Design review of the part shown in the three views and the two pictorial views. Dimensions are in mm from the part's minimum x, y and z. A direction names the side the tool comes from. Round coordinates to 2 decimals unless told otherwise and drop trailing zeros. Order: outer loops, then holes, each group sorted by start corner. A loop starts at its lowest first (then second) coordinate and runs counter-clockwise, first axis right, second up. Notation, with made-up numbers: (39, 85.25) - (93, 85.25) arc R20 cw to (93, 122.25) - close; hole circle Ø10 at (-11, 61). An arc over 180 degrees is marked (long way). Use CSV: the item, a comma, the result in double quotes.
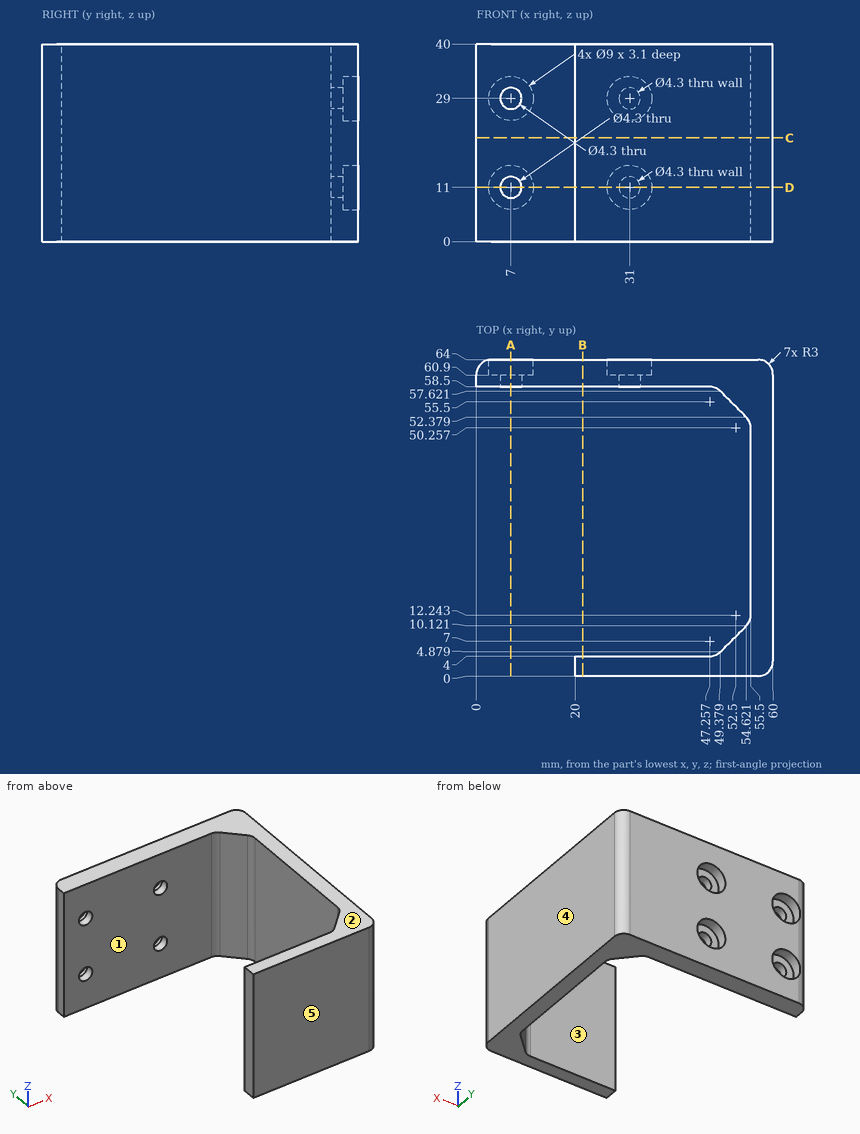
1) Insertion check: pin 1 Ø10 at (x, y) = (17.5, 54) entering from -Z; pin 2 Ø2.5 at (x, z) = (29.5, 10.5) entering from +Y; pin 3 Ø5 at (x, z) = (7, 11) entering from -Y; pin 4 Ø3 at (y, z) = (1.5, 26) entering from -X. Each pin has a flat end and moves straight along its axis. Give the tip position at first contact, or say it passes through.
Data:
pin 1,"stops at z = 0"
pin 2,"stops at y = 60.9"
pin 3,"stops at y = 58.5"
pin 4,"stops at x = 20"
2) We need section D-D (z = 11). Give the number of separate pieces and of enclosed holes in the cut face, then the cut area to 3 significant figures.
Data:
separate pieces,"3"
enclosed holes,"0"
area,"703 mm2"
3) The part is to be moulded in two halves that separate along Y. For the marked faces 3, 4 and 5, say which applies: +Y half, -Y half, draft (parallel to the pull), parting line (faces both ways), or undercut.
Data:
face 3,"undercut"
face 4,"draft"
face 5,"-Y half"
4) For the marked faces 1 and 2, list the 3-axis set-ups (+Z, -Z, +X, -X, +Y, -Y) from which the entire face can be reached by the end or side of a thin tool; tool diameter is ignored.
Data:
face 1,"+Z, -Z, -X"
face 2,"+Z, +X, -X, +Y, -Y"
5) We need section B-B (x = 21.5). Give the boundary of the cut face in (y, z).
Data:
outline,"(0, 0) - (4, 0) - (4, 40) - (0, 40) - close; (58.5, 0) - (64, 0) - (64, 40) - (58.5, 40) - close"
6) We need section C-C (z = 21). Give the boundary of the cut face in (x, y).
Data:
outline,"(0, 58.5) - (47.26, 58.5) arc R3 cw to (49.38, 57.62) - (54.62, 52.38) arc R3 cw to (55.5, 50.26) - (55.5, 12.24) arc R3 cw to (54.62, 10.12) - (49.38, 4.88) arc R3 cw to (47.26, 4) - (20, 4) - (20, 0) - (57, 0) arc R3 ccw to (60, 3) - (60, 61) arc R3 ccw to (57, 64) - (3, 64) arc R3 ccw to (0, 61) - close"
7) To check wall thickness, follow L1, parallel to Z at x = 7, y = 62.2; L2, parallel to Z at x = 7, y = 59.8; L3, parallel to Y at x = 44, z = 12.5. State the ranges of each line that lie inside material, in increasing order. Write a range as from..to.
Data:
L1,"z = 0..6.5, 15.5..24.5, 33.5..40"
L2,"z = 0..8.85, 13.15..26.85, 31.15..40"
L3,"y = 0..4, 58.5..64"
8) We need section A-A (x = 7). Give the boundary of the cut face in (y, z).
Data:
outline,"(58.5, 0) - (64, 0) - (64, 6.5) - (60.9, 6.5) - (60.9, 8.85) - (58.5, 8.85) - close; (58.5, 13.15) - (60.9, 13.15) - (60.9, 15.5) - (64, 15.5) - (64, 24.5) - (60.9, 24.5) - (60.9, 26.85) - (58.5, 26.85) - close; (58.5, 31.15) - (60.9, 31.15) - (60.9, 33.5) - (64, 33.5) - (64, 40) - (58.5, 40) - close"
